```python
from build123d import *

# Parameters (mm, degrees)
SKETCH1_W                                   = 80
SKETCH1_H                                   = 60
BOSS_EXTRUDE1_DEPTH                         = 100
CUT_EXTRUDE1_START                          = 5
SKETCH2_W                                   = 35
SKETCH2_H                                   = 55
CUT_EXTRUDE1_DEPTH                          = 95
SKETCH3_W                                   = 80
SKETCH3_H                                   = 5
BOSS_EXTRUDE2_DEPTH                         = 70
BOSS_EXTRUDE3_DEPTH                         = 10
SKETCH5_W                                   = 22.5
SKETCH5_H                                   = 2.5
SKETCH5_W_2                                 = 20
CUT_EXTRUDE2_DEPTH                          = 7.5
SKETCH6_W                                   = 35
SKETCH6_H                                   = 12
CUT_EXTRUDE4_DEPTH                          = 57.5
CUT_EXTRUDE6_REACH                          = 184.483
SKETCH7_R                                   = 4
SKETCH9_W                                   = 80
SKETCH9_H                                   = 50
BOSS_EXTRUDE4_DEPTH                         = 5
SKETCH11_W                                  = 75
SKETCH11_H                                  = 32.5
CUT_EXTRUDE7_DEPTH                          = 2
SKETCH13_W                                  = 7
SKETCH13_H                                  = 7
CUT_EXTRUDE8_DEPTH                          = 166.90660023
BOSS_EXTRUDE5_DEPTH                         = 10
SKETCH15_W                                  = 6
SKETCH15_H                                  = 4
BOSS_EXTRUDE6_DEPTH                         = 1
BOSS_EXTRUDE7_START                         = -2.5
SKETCH15_2_W                                = 6
SKETCH15_2_H                                = 4
BOSS_EXTRUDE7_DEPTH                         = 1
SKETCH17_W                                  = 6
SKETCH17_H                                  = 4
BOSS_EXTRUDE8_DEPTH                         = 1
SKETCH18_W                                  = 3
SKETCH18_H                                  = 4
CUT_EXTRUDE9_OLED_CABLE_DEPTH               = 154.430766146
SKETCH20_W                                  = 5
SKETCH20_H                                  = 5
CUT_EXTRUDE10_SOLENOID_WIRE_DEPTH           = 166.90660023
SKETCH21_W                                  = 5
SKETCH21_H                                  = 32
BOSS_EXTRUDE9_SOLENOID_SIDE_SUPPORT_DEPTH   = 13
SKETCH27_W                                  = 2.5
SKETCH27_H                                  = 50
BOSS_EXTRUDE13_SOLENOID_SECTION_WALLS_DEPTH = 15
SKETCH29_W                                  = 180
SKETCH29_H                                  = 5
BOSS_EXTRUDE9_GUIDE_DEPTH                   = 5
BOSS_EXTRUDE10_START                        = -80
SKETCH29_3_W                                = 180
SKETCH29_3_H                                = 5
BOSS_EXTRUDE10_GUIDE_DEPTH                  = 5


with BuildPart() as part:
    # Sketch1 → Boss-Extrude1 (new body)
    with BuildSketch(Plane(origin=(0, 0, 0), x_dir=(1, 0, 0), z_dir=(0, 1, 0))):
        with Locations((40, 30)):
            Rectangle(SKETCH1_W, SKETCH1_H)
    extrude(amount=BOSS_EXTRUDE1_DEPTH)

    # Sketch2 → Cut-Extrude1 (cut)
    with BuildSketch(Plane(origin=(0, 0, 0), x_dir=(1, 0, 0), z_dir=(0, 1, 0)).offset(CUT_EXTRUDE1_START)):
        with Locations((20, 30)):
            Rectangle(SKETCH2_W, SKETCH2_H)
        with Locations((60, 30)):
            Rectangle(SKETCH2_W, SKETCH2_H)
    extrude(amount=CUT_EXTRUDE1_DEPTH, mode=Mode.SUBTRACT)

    # Sketch3 → Boss-Extrude2 (add)
    with BuildSketch(Plane.XY):
        with Locations((40, 2.5)):
            Rectangle(SKETCH3_W, SKETCH3_H)
    extrude(amount=BOSS_EXTRUDE2_DEPTH)

    # Sketch4 → Boss-Extrude3 (add)
    with BuildSketch(Plane(origin=(0, 5, 0), x_dir=(1, 0, 0), z_dir=(0, 1, 0))):
        Polygon((80, 0), (77.5, 0), (77.5, -67.5), (42.5, -67.5), (42.5, 0), (37.5, 0), (37.5, -67.5), (2.5, -67.5), (2.5, 0), (0, 0), (0, -70), (80, -70), align=None)
    extrude(amount=BOSS_EXTRUDE3_DEPTH)

    # Sketch5 → Cut-Extrude2 (cut)
    with BuildSketch(Plane(origin=(0, 15, 0), x_dir=(1, 0, 0), z_dir=(0, 1, 0))):
        with Locations((18.75, -68.75)):
            Rectangle(SKETCH5_W, SKETCH5_H)
        with Locations((60, -68.75)):
            Rectangle(SKETCH5_W_2, SKETCH5_H)
    extrude(amount=-CUT_EXTRUDE2_DEPTH, mode=Mode.SUBTRACT)

    # Sketch6 → Cut-Extrude4 (cut)
    with BuildSketch(Plane.XY):
        with Locations((20, 11)):
            Rectangle(SKETCH6_W, SKETCH6_H)
        with Locations((60, 11)):
            Rectangle(SKETCH6_W, SKETCH6_H)
    extrude(amount=-CUT_EXTRUDE4_DEPTH, mode=Mode.SUBTRACT)

    # Sketch7 → Cut-Extrude6 (cut, up to next)
    with BuildSketch(Plane(origin=(0, 0, -60), x_dir=(-1, 0, 0), z_dir=(0, 0, -1)), mode=Mode.PRIVATE) as cut_extrude6_sk1:
        with Locations((-20, 11.5)):
            Circle(SKETCH7_R)
    cut_extrude6_tool1 = extrude(cut_extrude6_sk1.sketch, amount=-CUT_EXTRUDE6_REACH, mode=Mode.PRIVATE) & part.part
    # Sketch7 → Cut-Extrude6 (cut, up to next)
    with BuildSketch(Plane(origin=(0, 0, -60), x_dir=(-1, 0, 0), z_dir=(0, 0, -1)), mode=Mode.PRIVATE) as cut_extrude6_sk2:
        with Locations((-60, 11.5)):
            Circle(SKETCH7_R)
    cut_extrude6_tool2 = extrude(cut_extrude6_sk2.sketch, amount=-CUT_EXTRUDE6_REACH, mode=Mode.PRIVATE) & part.part
    add(cut_extrude6_tool1.solids().sort_by_distance((20, 11.5, -60))[0], mode=Mode.SUBTRACT)
    add(cut_extrude6_tool2.solids().sort_by_distance((60, 11.5, -60))[0], mode=Mode.SUBTRACT)

    # Sketch9 → Boss-Extrude4 (add)
    with BuildSketch(Plane(origin=(0, 0, 0), x_dir=(1, 0, 0), z_dir=(0, 1, 0))):
        with Locations((40, 85)):
            Rectangle(SKETCH9_W, SKETCH9_H)
    extrude(amount=BOSS_EXTRUDE4_DEPTH)

    # Sketch11 → Cut-Extrude7 (cut)
    with BuildSketch(Plane.XZ):
        with Locations((40, 53.75)):
            Rectangle(SKETCH11_W, SKETCH11_H)
    extrude(amount=-CUT_EXTRUDE7_DEPTH, mode=Mode.SUBTRACT)

    # Sketch13 → Cut-Extrude8 (cut, through all)
    with BuildSketch(Plane(origin=(0, 5, 0), x_dir=(1, 0, 0), z_dir=(0, 1, 0))):
        with Locations((20, -64)):
            Rectangle(SKETCH13_W, SKETCH13_H)
        with Locations((60, -64)):
            Rectangle(SKETCH13_W, SKETCH13_H)
    extrude(amount=-CUT_EXTRUDE8_DEPTH, mode=Mode.SUBTRACT)

    # Sketch14 → Boss-Extrude5 (add)
    with BuildSketch(Plane.XY):
        Polygon((25, 100), (26, 100), (26, 71), (54, 71), (54, 100), (55, 100), (55, 70), (54, 70), (26, 70), (25, 70), align=None)
    extrude(amount=BOSS_EXTRUDE5_DEPTH)

    # Sketch15 → Boss-Extrude6 (add)
    with BuildSketch(Plane.XY.offset(10)):
        with Locations((28, 72)):
            Rectangle(SKETCH15_W, SKETCH15_H)
        with Locations((52, 72)):
            Rectangle(SKETCH15_W, SKETCH15_H)
    extrude(amount=-BOSS_EXTRUDE6_DEPTH)

    # Sketch15<2> → Boss-Extrude7 (add)
    with BuildSketch(Plane.XY.offset(10).offset(BOSS_EXTRUDE7_START)):
        with Locations((28, 72)):
            Rectangle(SKETCH15_2_W, SKETCH15_2_H)
        with Locations((52, 72)):
            Rectangle(SKETCH15_2_W, SKETCH15_2_H)
    extrude(amount=-BOSS_EXTRUDE7_DEPTH)

    # Sketch17 → Boss-Extrude8 (add)
    with BuildSketch(Plane.XY.offset(10)):
        with Locations((28, 98)):
            Rectangle(SKETCH17_W, SKETCH17_H)
        with Locations((52, 98)):
            Rectangle(SKETCH17_W, SKETCH17_H)
    extrude(amount=-BOSS_EXTRUDE8_DEPTH)

    # Sketch18 → Cut-Extrude9 (OLED Cable) (cut, through all)
    with BuildSketch(Plane(origin=(0, 71, 0), x_dir=(1, 0, 0), z_dir=(0, 1, 0))):
        with Locations((40, -2)):
            Rectangle(SKETCH18_W, SKETCH18_H)
    extrude(amount=-CUT_EXTRUDE9_OLED_CABLE_DEPTH, mode=Mode.SUBTRACT)

    # Sketch20 → Cut-Extrude10 (Solenoid Wire) (cut, through all)
    with BuildSketch(Plane(origin=(0, 5, 0), x_dir=(1, 0, 0), z_dir=(0, 1, 0))):
        with Locations((60, 62.5)):
            Rectangle(SKETCH20_W, SKETCH20_H)
        with Locations((20, 62.5)):
            Rectangle(SKETCH20_W, SKETCH20_H)
    extrude(amount=-CUT_EXTRUDE10_SOLENOID_WIRE_DEPTH, mode=Mode.SUBTRACT)

    # Sketch21 → Boss-Extrude9 (Solenoid Side Support) (add)
    with BuildSketch(Plane(origin=(0, 5, 0), x_dir=(1, 0, 0), z_dir=(0, 1, 0))):
        with Locations((70, 76)):
            Rectangle(SKETCH21_W, SKETCH21_H)
        with Locations((50, 76)):
            Rectangle(SKETCH21_W, SKETCH21_H)
        with Locations((30, 76)):
            Rectangle(SKETCH21_W, SKETCH21_H)
        with Locations((10, 76)):
            Rectangle(SKETCH21_W, SKETCH21_H)
    extrude(amount=BOSS_EXTRUDE9_SOLENOID_SIDE_SUPPORT_DEPTH)

    # Sketch27 → Boss-Extrude13 (Solenoid Section Walls) (add)
    with BuildSketch(Plane(origin=(0, 5, 0), x_dir=(1, 0, 0), z_dir=(0, 1, 0))):
        with Locations((78.75, 85)):
            Rectangle(SKETCH27_W, SKETCH27_H)
        with Locations((1.25, 85)):
            Rectangle(SKETCH27_W, SKETCH27_H)
    extrude(amount=BOSS_EXTRUDE13_SOLENOID_SECTION_WALLS_DEPTH)

    # Sketch29 → Boss-Extrude9 (Guide) (add)
    with BuildSketch(Plane(origin=(80, 0, 0), x_dir=(0, 0, -1), z_dir=(1, 0, 0))):
        with Locations((20, 2.5)):
            Rectangle(SKETCH29_W, SKETCH29_H)
    extrude(amount=BOSS_EXTRUDE9_GUIDE_DEPTH)

    # Sketch29<3> → Boss-Extrude10 (Guide) (add)
    with BuildSketch(Plane(origin=(80, 0, 0), x_dir=(0, 0, -1), z_dir=(1, 0, 0)).offset(BOSS_EXTRUDE10_START)):
        with Locations((20, 2.5)):
            Rectangle(SKETCH29_3_W, SKETCH29_3_H)
    extrude(amount=-BOSS_EXTRUDE10_GUIDE_DEPTH)


solid = part.part
```
Geometry check sheet. Reference: the model listing, model coordinates, mm. A direction names the side the tool comes from. Coordinates: 2 decimals unless noted, no trailing zeros. Loops run counter-clockwise (first coordinate to the right, second up) from the corner with the lowest first, then second, coordinate; pieces in that order, holes last. Notation, with made-up numbers: (18.5, 33) - (76.5, 33) arc R28 cw to (76.5, 54) - close; hole circle Ø1 at (-29.75, -16.75). An arc over 180 degrees is marked (long way). One line per item, written item: value. Start each with the question number.
(1) Cross-section at C-C on z = 58. Enter the section's corners in (x, y).
(2) Cross-section at A-A on x = 9.5. Enter the section's corners in (y, z), plus the area to 3 significant figures.
(3) Cross-section at D-D on x = 60. Enter the section's corners in (y, z).
(4) Mould release check, pull along Z, two halves, no side actions. Record for faces 5 (the flat face through (30, 18, -76)), 6 (the flat face through (50, 11, -92)), 7 (the flat face through (20, 7, 67.5)): released by +Z, released by -Z, zero draft, split by the parting line, or undercut.
(5) Depth check by flat-ended pin: P1, Ø3, axis at x = 73, z = 17.5, coming from the +Y side; P2, Ø2.5, axis at x = 10, z = -79.5, coming from the +Y side; P3, Ø3, axis at y = 10, z = 69, coming from the -X side. Enter the tip coordinate at first touch or a pass-through.
(6) Material ranges on line 1 (X direction, y = 17, z = -50); line 2 (X direction, y = 11, z = -59); line 3 (Z direction, x = 45, y = 91), recorded low to high. Write a range as [from, to].
(7) Tool access check on faces 1 (the flat face through (20, 58, -2.5)), 2 (the flat face through (22.5, 3, -62)), 3 (the flat face through (72.5, 11, -76)), 4 (the flat face through (40, 70, 5)). Record the directions out of +Z, -Z, +X, -X, +Y, -Y that give a thin tool (end or side, any length) a straight path to the whole face; none if there is none.
(8) Cross-section at B-B on y = 80. Enter the section's corners in (x, z), plus the area to 3 significant figures.
Results below:
1. outline: (-5, 0) - (2.5, 0) - (2.5, 2) - (77.5, 2) - (77.5, 0) - (85, 0) - (85, 5) - (80, 5) - (80, 15) - (77.5, 15) - (77.5, 5) - (42.5, 5) - (42.5, 15) - (37.5, 15) - (37.5, 5) - (2.5, 5) - (2.5, 15) - (0, 15) - (0, 5) - (-5, 5) - close
2. outline: (0, -110) - (5, -110) - (5, -92) - (18, -92) - (18, -60) - (100, -60) - (100, -57.5) - (5, -57.5) - (5, 67.5) - (7.5, 67.5) - (7.5, 70) - (2, 70) - (2, 37.5) - (0, 37.5) - close; (17, -2.5) - (100, -2.5) - (100, 0) - (17, 0) - close
2. area: 1,700 mm2
3. outline: (0, -110) - (5, -110) - (5, -65) - (0, -65) - close; (0, -60) - (7.5, -60) - (7.5, -57.5) - (5, -57.5) - (5, 60.5) - (2, 60.5) - (2, 37.5) - (0, 37.5) - close; (2, 67.5) - (7.5, 67.5) - (7.5, 70) - (2, 70) - close; (15.5, -60) - (100, -60) - (100, -57.5) - (15.5, -57.5) - close; (17, -2.5) - (100, -2.5) - (100, 0) - (17, 0) - close
4. face 5: zero draft
4. face 6: released by -Z
4. face 7: undercut
5. P1: stops at y = 5
5. P2: stops at y = 18
5. P3: stops at x = 0
6. line 1: x = [0, 2.5], [37.5, 42.5], [77.5, 80]
6. line 2: x = [0, 16.03], [23.97, 56.03], [63.97, 80]
6. line 3: z = [-60, -57.5], [-2.5, 0]
7. face 1: +Y
7. face 2: +Y, -Y
7. face 3: -Z, +Y
7. face 4: +Z, +X, -X
8. outline: (0, -60) - (80, -60) - (80, 0) - (55, 0) - (55, 10) - (54, 10) - (54, 0) - (26, 0) - (26, 10) - (25, 10) - (25, 0) - (0, 0) - close; hole (2.5, -57.5) - (37.5, -57.5) - (37.5, -2.5) - (2.5, -2.5) - close; hole (42.5, -57.5) - (77.5, -57.5) - (77.5, -2.5) - (42.5, -2.5) - close
8. area: 970 mm2
